Autodesk Inventor part; units mm, degrees
ref_plane "YZ Plane" through (0, 0, 0) normal (1, 0, 0) x (0, 1, 0)
ref_plane "XZ Plane" through (0, 0, 0) normal (0, 1, 0) x (-1, 0, 0)
ref_plane "XY Plane" through (0, 0, 0) normal (0, 0, 1) x (1, 0, 0)
sketch "スケッチ1" plane through (0, 0, 0) normal (0, 0, 1) x (1, 0, 0)
  line L0 (0, -31) -> (0, -46)
  line L1 (0, -31) -> (-140, -31)
  line L2 (-140, -46) -> (-140, -31)
  line L3 (0, -46) -> (-140, -46)
  line L4 (-30, 15) -> (-110, 15)
  line L5 (-110, 15) -> (-110, -46)
  line L6 (-110, -46) -> (-30, -46)
  line L7 (-30, -46) -> (-30, 15)
  line L8 (0, 15) -> (0, 0)
  line L9 (0, 15) -> (-140, 15)
  line L10 (-140, 0) -> (-140, 15)
  line L11 (0, 0) -> (-140, 0)
  circle A0 centre (-37.5, 7.5) radius 1.6
  circle A1 centre (-102.5, 7.5) radius 1.6
  circle A2 centre (-37.5, -38.5) radius 1.6
  circle A3 centre (-102.5, -38.5) radius 1.6
  dimension "d1" = 80
  dimension "d15" = 30
extrude "押し出し1" add sketch "スケッチ1" along normal blind 3 contours L7 L3 L5 L1 | L1 L5 L11 L7 | L11 L5 L4 L7 | A0 | A1 | A2 | A3
sketch "スケッチ2" plane through (0, 0, 3) normal (0, 0, 1) x (1, 0, 0)
  line L0 (-110, -46) -> (-30, -46)
  line L1 (-30, 15) -> (-110, 15)
  line L2 (-30, -46) -> (-30, 15)
  line L3 (-110, 15) -> (-110, -46)
  point P0 (0, 0)
  point P1 (-37.5, 7.5)
  point P2 (-37.5, -38.5)
  point P3 (-102.5, -38.5)
  point P4 (-102.5, 7.5)
  dimension "d4" = 7.5
  dimension "d5" = 7.5
  dimension "d6" = 7.5
  dimension "d7" = 7.5
hole "穴1" at (-37.5, 7.5, 3) at (-37.5, -38.5, 3) at (-102.5, -38.5, 3) at (-102.5, 7.5, 3) direction (0, 0, -1) diameter 2.459 end through all
sketch "スケッチ3" plane through (0, 0, 3) normal (0, 0, 1) x (1, 0, 0)
  line L0 (-52, -28) -> (-66, -28)
  line L1 (-69, -28) -> (-69, -31)
  line L2 (-52, -31) -> (-66, -31)
  line L3 (-49, -28) -> (-49, -31)
  line L4 (-30, -46) -> (-30, 15)
  line L5 (-110, -46) -> (-30, -46)
  arc A0 (-69, -31) -> (-66, -31) centre (-67.5, -31) ccw
  arc A1 (-52, -31) -> (-49, -31) centre (-50.5, -31) ccw
  arc A2 (-66, -28) -> (-69, -28) centre (-67.5, -28) ccw
  arc A3 (-49, -28) -> (-52, -28) centre (-50.5, -28) ccw
  circle A4 centre (-59, -25) radius 1.6
  point P0 (0, 0)
  point P1 (-59, -28)
  dimension "d16" = 19
  dimension "d17" = 15
  dimension "d18" = 3
  dimension "d19" = 20
  dimension "d21" = 3
  dimension "d32" = 3
  dimension "d33" = 3.2
extrude "押し出し2" cut sketch "スケッチ3" against normal blind 3
ref_plane "作業平面1" through (-110, -15.5, 0) normal (0, 1, 0) x (1, 0, 0)
mirror "ミラー1" about plane through (-110, -15.5, 0) normal (0, 1, 0) of "押し出し2"
pattern_linear "矩形状パターン1" count 2 spacing 34 along (-1, 0, 0) of "押し出し2", "ミラー1"
properties part number "plate2" material "アルミニウム 2014-T4"
Verification items for the finished model (mm, model axes). Coordinates: 2 decimals unless noted, no trailing zeros. Write each loop counter-clockwise with the first axis right and the second up, starting at its lowest first coordinate (ties: lowest second). Pieces come first, ordered by that corner, then holes. Notation, with made-up numbers: M 77,53 L 113,53 A11 ccw 113,67 Z; hole C 50.5,40.25 d1. An arc over 180 degrees is marked long. One line per item, written item: value.
Item 1: Gauge pin test, flat end, axial feed: pin 1 Ø1.9 at (x, y) = (-93, -25) entering from +Z. Record the tip position at first contact, or that the pin passes through.
Check sheet entries:
pin 1: passes through
Item 2: Section check D-D, the plane z = 1.4. State how many separate pieces and enclosed holes the cut face has, plus the area to 3 significant figures.
Check sheet entries:
separate pieces: 1
enclosed holes: 12
area: 4,530 mm^2
Item 3: Section check C-C, the plane x = -93. Record the boundary of the cut face in (y, z).
Check sheet entries:
outline: M -46,0 L -31,0 L -31,3 L -46,3 Z; M -28,0 L -26.6,0 L -26.6,3 L -28,3 Z; M -23.4,0 L -7.6,0 L -7.6,3 L -23.4,3 Z; M -4.4,0 L -3,0 L -3,3 L -4.4,3 Z; M 0,0 L 15,0 L 15,3 L 0,3 Z
Item 4: Scan lines: line 1 along Y through (x, z) = (-93, 1.25); line 2 along Y through (x, z) = (-88, 0.8); line 3 along X through (y, z) = (7.5, 2.05). Record each from-to range of solid material in increasing order.
Check sheet entries:
line 1: y = -46 to -31, -28 to -26.6, -23.4 to -7.6, -4.4 to -3, 0 to 15
line 2: y = -46 to -31, -28 to -3, 0 to 15
line 3: x = -110 to -103.73, -101.27 to -38.73, -36.27 to -30
Item 5: Section check A-A, the plane x = -64.5. Record the boundary of the cut face in (y, z), plus the area to 3 significant figures.
Check sheet entries:
outline: M -46,0 L -31,0 L -31,3 L -46,3 Z; M -28,0 L -3,0 L -3,3 L -28,3 Z; M 0,0 L 15,0 L 15,3 L 0,3 Z
area: 165 mm^2
Item 6: Mould release check, pull along Y, two halves, no side actions. Record for faces 1 (the flat face through (-69, 15, 1)), 2 (the flat face through (-103, -1, 2)): pulls with the +Y half, pulls with the -Y half, needs draft (parallel to the pull), parting line crosses it, or undercut.
Check sheet entries:
face 1: pulls with the +Y half
face 2: undercut
Item 7: Section check B-B, the plane y = 7.5. Record the boundary of the cut face in (x, z), plus the area to 3 significant figures.
Check sheet entries:
outline: M -110,0 L -103.73,0 L -103.73,3 L -110,3 Z; M -101.27,0 L -38.73,0 L -38.73,3 L -101.27,3 Z; M -36.27,0 L -30,0 L -30,3 L -36.27,3 Z
area: 225 mm^2
